Here's how the part is built. I have some questions about the finished solid (model axes, mm). A direction names the side the tool comes from. Round coordinates to 2 decimals unless told otherwise and drop trailing zeros. Order: outer loops, then holes, each group sorted by start corner. A loop starts at its lowest first (then second) coordinate and runs counter-clockwise, first axis right, second up.
Autodesk Inventor part; units mm, degrees
ref_plane "작업 평면1" through (94.5, 0, 0) normal (1, 0, 0) x (0, 0, -1)
ref_plane "YZ Plane" through (0, 0, 0) normal (1, 0, 0) x (0, 1, 0)
ref_plane "XZ Plane" through (0, 0, 0) normal (0, 1, 0) x (-1, 0, 0)
sketch "스케치1" plane through (0, 0, 0) normal (0, 0, 1) x (1, 0, 0)
  line L0 (0, 0) -> (120, 0)
  line L1 (120, 0) -> (120, 75)
  line L2 (120, 75) -> (0, 75)
  line L3 (0, 75) -> (0, 0)
  dimension "d0" = 120
  dimension "d1" = 75
extrude "돌출1" add sketch "스케치1" along normal blind 9
sketch "스케치2" plane through (0, 0, 9) normal (0, 0, 1) x (1, 0, 0)
  line L0 (25.5, 59.5) -> (94.5, 59.5)
  line L1 (94.5, 59.5) -> (94.5, 15.5)
  line L2 (94.5, 15.5) -> (25.5, 15.5)
  line L3 (25.5, 15.5) -> (25.5, 59.5)
  line L4 (0, 75) -> (0, 0)
  line L5 (0, 0) -> (120, 0)
  dimension "d4" = 44
  dimension "d5" = 69
  dimension "d6" = 25.5
  dimension "d7" = 15.5
ref_plane "작업 평면1" through (94.5, 0, 0) normal (1, 0, 0) x (0, 0, -1)
sketch "스케치3" plane through (94.5, 0, 0) normal (1, 0, 0) x (0, 0, -1)
  line L0 (-9, 0) -> (-9, 75)
  line L1 (-9, 59.5) -> (-9, 15.5)
  line L2 (-9, 59.5) -> (-17.9999, 15.5)
  line L3 (-17.9999, 15.5) -> (-9, 15.5)
  point P0 (0, 0)
  dimension "d9" = 11.56
  dimension "d10" = 90
extrude "돌출2" add sketch "스케치3" against normal blind 69
fillet "모깎기1" radius 10 1 edges at (120, 37.5, 9)
fillet "모깎기2" radius 10 1 edges at (0, 37.5, 9)
properties part number "스위치"
1. I'm going to push flat-ended pins straight in: P1, Ø10, axis at y = 42.5, z = 11.5, coming from the +X side; P2, Ø2.5, axis at x = 66.5, z = 12, coming from the -Y side; P3, Ø8, axis at x = 75.5, y = 66.5, coming from the +Z side. Where does each tip first touch, or does it pass through?
Evaluation:
P1: stops at x = 116.66
P2: stops at y = 15.5
P3: stops at z = 9
2. On a 3-axis mill with a long thin cutter (end or side, diameter ignored), from which of +Z, -Z, +X, -X, +Y, -Y can I reach the whole of each face in a straight line? I mean faces 1 (the flat face through (59, 0, 4)), 2 (the flat face through (61, 75, 4)), 3 (the flat face through (94.5, 28, 12)), 4 (the flat face through (60, 15.5, 14)), 5 (the flat face through (25.5, 28, 12)). Say none if no direction works.
Evaluation:
face 1: +Z, -Z, +X, -X, -Y
face 2: +Z, -Z, +X, -X, +Y
face 3: +Z, +X, +Y, -Y
face 4: +Z, +X, -X, -Y
face 5: +Z, -X, +Y, -Y
3. If we section it at C-C, the plane z = 11.5: Write out the boundary of the cut face in (x, y), and give its area (3 significant figures).
Evaluation:
outline: (25.5, 15.5) - (94.5, 15.5) - (94.5, 47.28) - (25.5, 47.28) - close
area: 2,190 mm2
4. If we section it at B-B, the plane y = 28: Write out the boundary of the cut face in (x, z).
Evaluation:
outline: (0, 0) - (120, 0) arc R10 ccw to (110.05, 9) - (94.5, 9) - (94.5, 15.44) - (25.5, 15.44) - (25.5, 9) - (9.95, 9) arc R10 ccw to start
5. I need wall thicknesses on probe 1 along X at (y, z) = (23, 12.5); probe 2 along Z at (x, y) = (95, 12.5); probe 3 along X at (y, z) = (68.5, 7.25). Which ranges of each line are inside material? Lowest first, please.
Evaluation:
probe 1: x = 25.5 to 94.5
probe 2: z = 0 to 9
probe 3: x = 4.3 to 115.7
6. If we section it at A-A, the plane x = 34.5: Write out the boundary of the cut face in (y, z).
Evaluation:
outline: (0, 0) - (75, 0) - (75, 9) - (59.5, 9) - (15.5, 18) - (15.5, 9) - (0, 9) - close
7. If we section it at D-D, the plane y = 46.5: Write out the boundary of the cut face in (x, z).
Evaluation:
outline: (0, 0) - (120, 0) arc R10 ccw to (110.05, 9) - (94.5, 9) - (94.5, 11.66) - (25.5, 11.66) - (25.5, 9) - (9.95, 9) arc R10 ccw to start
